Read the model definition and answer for the solid it produces. Units are mm, in the model's axes. Face numbers are marked on the shaded views. Give positions to 0.01 mm unless a question says otherwise; leave off trailing zeros. Write each loop counter-clockwise with the first axis right and the second up, starting at its lowest first coordinate (ties: lowest second). Pieces come first, ordered by that corner, then holes. Notation, with made-up numbers: (39.5, 60) - (48.5, 60) arc R19 ccw to (48.5, 85) - close; hole circle Ø9 at (63, 69). An arc over 180 degrees is marked (long way). Use CSV: the item, a comma, the result in double quotes. Start each with the question number.
from build123d import *

# Parameters (mm, degrees)
SKETCH1_R           = 14
SKETCH1_R_2         = 4.5
BOSS_EXTRUDE1_DEPTH = 3
CUT_EXTRUDE1_DEPTH  = 0.5
FILLET1_R           = 0.2


with BuildPart() as part:
    # Sketch1 → Boss-Extrude1 (new body)
    with BuildSketch(Plane(origin=(0, 0, 0), x_dir=(1, 0, 0), z_dir=(0, 1, 0))):
        with Locations(Location((0, 0, 0), (0, 0, 270))):
            Circle(SKETCH1_R)
        with Locations(Location((0, 0, 0), (0, 0, 270))):
            Circle(SKETCH1_R_2, mode=Mode.SUBTRACT)
    extrude(amount=BOSS_EXTRUDE1_DEPTH)

    # Sketch2 → Cut-Extrude1 (cut)
    with BuildSketch(Plane(origin=(0, 3, 0), x_dir=(1, 0, 0), z_dir=(0, 1, 0))):
        with BuildLine():
            Line((-2.165063509, 6.75), (-4.165063509, 10.214101615))
            Line((-4.165063509, 10.214101615), (-3.732050808, 10.464101615))
            Line((-3.732050808, 10.464101615), (-1.732050808, 7))
            ThreePointArc((-1.732050808, 7), (0, 6), (1.732050808, 7))
            Line((1.732050808, 7), (3.732050808, 10.464101615))
            Line((3.732050808, 10.464101615), (4.165063509, 10.214101615))
            Line((4.165063509, 10.214101615), (2.165063509, 6.75))
            ThreePointArc((2.165063509, 6.75), (0, 5.5), (-2.165063509, 6.75))
        make_face()
        with BuildLine():
            Line((5.196152423, 5), (7.196152423, 8.464101615))
            Line((7.196152423, 8.464101615), (6.763139721, 8.714101615))
            Line((6.763139721, 8.714101615), (4.763139721, 5.25))
            ThreePointArc((4.763139721, 5.25), (4.763139721, 2.75), (6.92820323, 1.5))
            Line((6.92820323, 1.5), (10.92820323, 1.5))
            Line((10.92820323, 1.5), (10.92820323, 2))
            Line((10.92820323, 2), (6.92820323, 2))
            ThreePointArc((6.92820323, 2), (5.196152423, 3), (5.196152423, 5))
        make_face()
        with BuildLine():
            Line((6.92820323, -2), (10.92820323, -2))
            Line((10.92820323, -2), (10.92820323, -1.5))
            Line((10.92820323, -1.5), (6.92820323, -1.5))
            ThreePointArc((6.92820323, -1.5), (4.763139721, -2.75), (4.763139721, -5.25))
            Line((4.763139721, -5.25), (6.763139721, -8.714101615))
            Line((6.763139721, -8.714101615), (7.196152423, -8.464101615))
            Line((7.196152423, -8.464101615), (5.196152423, -5))
            ThreePointArc((5.196152423, -5), (5.196152423, -3), (6.92820323, -2))
        make_face()
        with BuildLine():
            Line((1.732050808, -7), (3.732050808, -10.464101615))
            Line((3.732050808, -10.464101615), (4.165063509, -10.214101615))
            Line((4.165063509, -10.214101615), (2.165063509, -6.75))
            ThreePointArc((2.165063509, -6.75), (0, -5.5), (-2.165063509, -6.75))
            Line((-2.165063509, -6.75), (-4.165063509, -10.214101615))
            Line((-4.165063509, -10.214101615), (-3.732050808, -10.464101615))
            Line((-3.732050808, -10.464101615), (-1.732050808, -7))
            ThreePointArc((-1.732050808, -7), (0, -6), (1.732050808, -7))
        make_face()
        with BuildLine():
            Line((-5.196152423, -5), (-7.196152423, -8.464101615))
            Line((-7.196152423, -8.464101615), (-6.763139721, -8.714101615))
            Line((-6.763139721, -8.714101615), (-4.763139721, -5.25))
            ThreePointArc((-4.763139721, -5.25), (-4.763139721, -2.75), (-6.92820323, -1.5))
            Line((-6.92820323, -1.5), (-10.92820323, -1.5))
            Line((-10.92820323, -1.5), (-10.92820323, -2))
            Line((-10.92820323, -2), (-6.92820323, -2))
            ThreePointArc((-6.92820323, -2), (-5.196152423, -3), (-5.196152423, -5))
        make_face()
        with BuildLine():
            Line((-6.92820323, 2), (-10.92820323, 2))
            Line((-10.92820323, 2), (-10.92820323, 1.5))
            Line((-10.92820323, 1.5), (-6.92820323, 1.5))
            ThreePointArc((-6.92820323, 1.5), (-4.763139721, 2.75), (-4.763139721, 5.25))
            Line((-4.763139721, 5.25), (-6.763139721, 8.714101615))
            Line((-6.763139721, 8.714101615), (-7.196152423, 8.464101615))
            Line((-7.196152423, 8.464101615), (-5.196152423, 5))
            ThreePointArc((-5.196152423, 5), (-5.196152423, 3), (-6.92820323, 2))
        make_face()
    extrude(amount=-CUT_EXTRUDE1_DEPTH, mode=Mode.SUBTRACT)

    # Fillet1
    fillet1_edges = [part.edges().sort_by_distance(p)[0] for p in [
        (0, 0, -14),
        (0, 3, -14),
        (0, 0, -4.5),
        (0, 3, -4.5),
    ]]
    fillet(fillet1_edges, radius=FILLET1_R)


solid = part.part
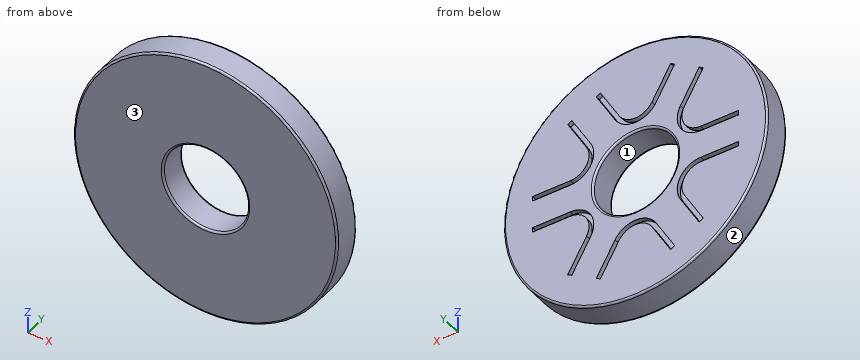
(1) Given P1, Ø1.5, axis at y = 1, z = 2.5, coming from the +X side; P2, Ø1, axis at x = 2.5, y = 1.5, coming from the -Z side; P3, Ø1, axis at y = 1, z = -5.5, coming from the -X side, each flat-ended and moving along its own axis, determine where each tip first touches the part or whether it passes through.
(2) Consider probe 1 along X at (y, z) = (2.1, 0); probe 2 along X at (y, z) = (2.75, -6.5); probe 3 along Z at (x, y) = (8.75, 2.2). Determine where each line is inside the solid, lowest interval first.
(3) For a pull along X with two mould halves and no side action, classify the marked faces 1, 2 and 3 as pulls with the +X half, pulls with the -X half, needs draft (parallel to the pull), parting line crosses it, or undercut.
(4) The part is cut by section B-B on z = 0. Write down the section's boundary in (x, y), plus the area to 3 significant figures.
(5) The part is cut by section A-A on x = 0. Write down the section's boundary in (y, z), plus the area to 3 significant figures.
(6) The part is cut by section C-C on y = 1.4. Write down the section's boundary in (x, z).
Reported:
1,P1,"x = 13.89"
1,P2,"z = -13.86"
1,P3,"x = -13.08"
2,probe 1,"-14 to -4.5, 4.5 to 14"
2,probe 2,"-12.4 to -6.06, -5.48 to -2, -1.32 to 1.32, 2 to 5.48, 6.06 to 12.4"
2,probe 3,"-10.93 to 10.93"
3,face 1,"undercut"
3,face 2,"parting line crosses it"
3,face 3,"needs draft"
4,outline,"(-14, 0.2) arc R0.2 ccw to (-13.8, 0) - (-4.7, 0) arc R0.2 ccw to (-4.5, 0.2) - (-4.5, 2.8) arc R0.2 ccw to (-4.7, 3) - (-13.8, 3) arc R0.2 ccw to (-14, 2.8) - close; (4.5, 0.2) arc R0.2 ccw to (4.7, 0) - (13.8, 0) arc R0.2 ccw to (14, 0.2) - (14, 2.8) arc R0.2 ccw to (13.8, 3) - (4.7, 3) arc R0.2 ccw to (4.5, 2.8) - close"
4,area,"56.9 mm²"
5,outline,"(0, -13.8) arc R0.2 ccw to (0.2, -14) - (2.8, -14) arc R0.2 ccw to (3, -13.8) - (3, -6) - (2.5, -6) - (2.5, -5.5) - (3, -5.5) - (3, -4.7) arc R0.2 ccw to (2.8, -4.5) - (0.2, -4.5) arc R0.2 ccw to (0, -4.7) - close; (0, 4.7) arc R0.2 ccw to (0.2, 4.5) - (2.8, 4.5) arc R0.2 ccw to (3, 4.7) - (3, 5.5) - (2.5, 5.5) - (2.5, 6) - (3, 6) - (3, 13.8) arc R0.2 ccw to (2.8, 14) - (0.2, 14) arc R0.2 ccw to (0, 13.8) - close"
5,area,"56.4 mm²"
6,outline,"circle Ø28 at (0, 0); hole circle Ø9 at (0, 0)"
